Design review of the part built by this model. Coordinates are the model's own, in mm. Face numbers are marked on the shaded views. Round coordinates to 2 decimals unless told otherwise and drop trailing zeros. Order: outer loops, then holes, each group sorted by start corner. A loop starts at its lowest first (then second) coordinate and runs counter-clockwise, first axis right, second up. Notation, with made-up numbers: (28.25, 63) - (38.25, 63) arc R26 cw to (38.25, 93) - close; hole circle Ø3 at (53, 48.5). An arc over 180 degrees is marked (long way). Write item = value, one per line.
from build123d import *

# Parameters (mm, degrees)
F2_W = 5
F2_H = 5


with BuildPart() as f3:
    # F3: sweep along a path in F0
    with BuildLine(Plane.XZ) as f3_path:
        Line((-33, 10), (-33, -10))
        Line((-33, -10), (33, -10))
        Line((33, -10), (33, 10))
    # F2 (on plane+point) → F3 (sweep)
    with BuildSketch(Plane.XY.offset(10)):
        with Locations((-33, 0)):
            Rectangle(F2_W, F2_H)
    sweep(path=f3_path.line, transition=Transition.RIGHT)


solid = f3.part
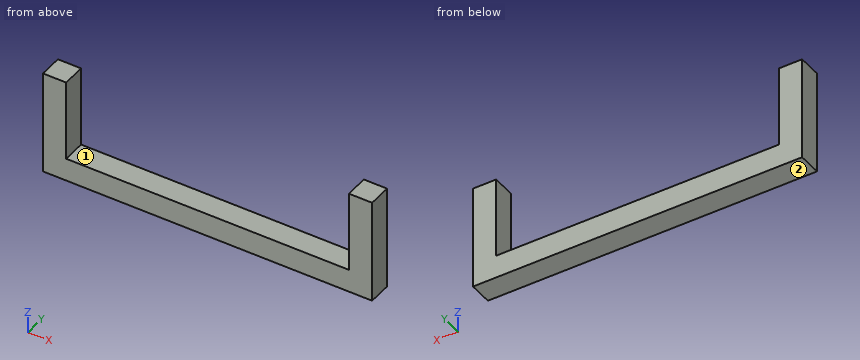
Item 1: Take a section at C-C, the plane x = 13. State the section outline as (y, z) points.
Data:
outline = (-2.5, -12.5) - (2.5, -12.5) - (2.5, -7.5) - (-2.5, -7.5) - close
Item 2: Take a section at B-B, the plane y = 0.1. State the section outline as (x, z) points, and give its area (3 significant figures).
Data:
outline = (-35.5, -12.5) - (35.5, -12.5) - (35.5, 10) - (30.5, 10) - (30.5, -7.5) - (-30.5, -7.5) - (-30.5, 10) - (-35.5, 10) - close
area = 530 mm2
Item 3: The part is to be moulded in two halves that separate along X. For the marked faces 1 and 2, say which applies: +X half, -X half, draft (parallel to the pull), parting line (faces both ways), or undercut.
Data:
face_1 = undercut
face_2 = draft
Item 4: Take a section at A-A, the plane z = 1. State the section outline as (x, y) points, and give its area (3 significant figures).
Data:
outline = (-35.5, -2.5) - (-30.5, -2.5) - (-30.5, 2.5) - (-35.5, 2.5) - close; (30.5, -2.5) - (35.5, -2.5) - (35.5, 2.5) - (30.5, 2.5) - close
area = 50.0 mm2
Item 5: Insertion check: P1, Ø5, axis at x = -26.5, z = 1, coming from the -Y side; P2, Ø2.5, axis at x = -2, y = 0, coming from the +Z side. Each pin has a flat end and moves straight along its axis. Give the tip position at first contact, or say it passes through.
Data:
P1 = through
P2 = -7.5
Item 6: For line 1 along X through (y, z) = (1.65, 7.25); line 2 along Z through (x, y) = (-11, 0.5), list the stretches that pass through material, from the lowest coordinate up. Write a range as [from, to].
Data:
line_1 = [-35.5, -30.5], [30.5, 35.5]
line_2 = [-12.5, -7.5]
